```python
from build123d import *

# Parameters (mm, degrees)
ESQUISSE1_W             = 45
ESQUISSE1_H             = 45
BOSS_EXTRU_1_DEPTH      = 5
BOSS_EXTRU_2_DEPTH      = 20
BOSS_EXTRU_3_DEPTH      = 12
CONG_1_R                = 10
ESQUISSE4_W             = 4
ESQUISSE4_H             = 31.383485478
ENL_V_MAT_EXTRU_1_DEPTH = 1
ESQUISSE6_W             = 4
ESQUISSE6_H             = 28.242544177
ENL_V_MAT_EXTRU_2_DEPTH = 1
CONG_2_R                = 1
CONG_3_R                = 0.5


with BuildPart() as part:
    # Esquisse1 → Boss.-Extru.1 (new body)
    with BuildSketch(Plane.XY):
        Rectangle(ESQUISSE1_W, ESQUISSE1_H)
        with BuildLine():
            Line((14.767944635, 16.889264979), (16.889264979, 14.767944635))
            ThreePointArc((16.889264979, 14.767944635), (17.182158197, 14.060837854), (16.889264979, 13.353731073))
            Line((16.889264979, 13.353731073), (15.475051416, 11.93951751))
            ThreePointArc((15.475051416, 11.93951751), (14.828187526, 11.496881699), (14.060837854, 11.656674798))
            Line((14.060837854, 11.656674798), (11.798096154, 13.919416498))
            ThreePointArc((11.798096154, 13.919416498), (11.505202935, 14.626523279), (11.798096154, 15.33363006))
            Line((11.798096154, 15.33363006), (13.353731073, 16.889264979))
            ThreePointArc((13.353731073, 16.889264979), (14.060837854, 17.182158197), (14.767944635, 16.889264979))
        make_face(mode=Mode.SUBTRACT)
        with BuildLine():
            Line((11.93951751, -15.475051416), (13.353731073, -16.889264979))
            ThreePointArc((13.353731073, -16.889264979), (14.060837854, -17.182158197), (14.767944635, -16.889264979))
            Line((14.767944635, -16.889264979), (16.889264979, -14.767944635))
            ThreePointArc((16.889264979, -14.767944635), (17.182158197, -14.060837854), (16.889264979, -13.353731073))
            Line((16.889264979, -13.353731073), (15.33363006, -11.798096154))
            ThreePointArc((15.33363006, -11.798096154), (14.626523279, -11.505202935), (13.919416498, -11.798096154))
            Line((13.919416498, -11.798096154), (11.656674798, -14.060837854))
            ThreePointArc((11.656674798, -14.060837854), (11.496881699, -14.828187526), (11.93951751, -15.475051416))
        make_face(mode=Mode.SUBTRACT)
        with BuildLine():
            Line((-15.475051416, -11.93951751), (-16.889264979, -13.353731073))
            ThreePointArc((-16.889264979, -13.353731073), (-17.182158197, -14.060837854), (-16.889264979, -14.767944635))
            Line((-16.889264979, -14.767944635), (-14.767944635, -16.889264979))
            ThreePointArc((-14.767944635, -16.889264979), (-14.060837854, -17.182158197), (-13.353731073, -16.889264979))
            Line((-13.353731073, -16.889264979), (-11.798096154, -15.33363006))
            ThreePointArc((-11.798096154, -15.33363006), (-11.505202935, -14.626523279), (-11.798096154, -13.919416498))
            Line((-11.798096154, -13.919416498), (-14.060837854, -11.656674798))
            ThreePointArc((-14.060837854, -11.656674798), (-14.828187526, -11.496881699), (-15.475051416, -11.93951751))
        make_face(mode=Mode.SUBTRACT)
        with BuildLine():
            Line((-11.93951751, 15.475051416), (-13.353731073, 16.889264979))
            ThreePointArc((-13.353731073, 16.889264979), (-14.060837854, 17.182158197), (-14.767944635, 16.889264979))
            Line((-14.767944635, 16.889264979), (-16.889264979, 14.767944635))
            ThreePointArc((-16.889264979, 14.767944635), (-17.182158197, 14.060837854), (-16.889264979, 13.353731073))
            Line((-16.889264979, 13.353731073), (-15.33363006, 11.798096154))
            ThreePointArc((-15.33363006, 11.798096154), (-14.626523279, 11.505202935), (-13.919416498, 11.798096154))
            Line((-13.919416498, 11.798096154), (-11.656674798, 14.060837854))
            ThreePointArc((-11.656674798, 14.060837854), (-11.496881699, 14.828187526), (-11.93951751, 15.475051416))
        make_face(mode=Mode.SUBTRACT)
    extrude(amount=BOSS_EXTRU_1_DEPTH)

    # Esquisse2 → Boss.-Extru.2 (add)
    with BuildSketch(Plane.XY.offset(5)):
        Polygon((-1, 22.5), (-1, 1), (-22.5, 1), (-22.5, -1), (-1, -1), (-1, -22.5), (1, -22.5), (1, -1), (22.5, -1), (22.5, 1), (1, 1), (1, 22.5), align=None)
    extrude(amount=BOSS_EXTRU_2_DEPTH)

    # Esquisse3 → Boss.-Extru.3 (add)
    with BuildSketch(Plane(origin=(0, 0, 0), x_dir=(-1, 0, 0), z_dir=(0, 0, -1))):
        Polygon((-20.68287335, 0.883883476), (-0.883883476, 20.68287335), (20.68287335, -0.883883476), (0.883883476, -20.68287335), align=None)
    extrude(amount=BOSS_EXTRU_3_DEPTH)

    # Congé1
    cong_1_edges = [part.edges().sort_by_distance(p)[0] for p in [
        (0, 22.5, 25),
        (-22.5, 0, 25),
        (0, -22.5, 25),
        (22.5, 0, 25),
    ]]
    fillet(cong_1_edges, radius=CONG_1_R)

    # Esquisse4 → Enlèv. mat.-Extru.1 (cut)
    with BuildSketch(Plane(origin=(10.783378413, 10.783378413, 0), x_dir=(0, 0, -1), z_dir=(0.7071067811865475, 0.7071067811865477, 0))):
        with Locations((2, -1.691742739)):
            Rectangle(ESQUISSE4_W, ESQUISSE4_H)
    extrude(amount=-ENL_V_MAT_EXTRU_1_DEPTH, mode=Mode.SUBTRACT)

    # Esquisse6 → Enlèv. mat.-Extru.2 (cut)
    with BuildSketch(Plane(origin=(-10.783378413, -10.783378413, 0), x_dir=(0, 0, 1), z_dir=(-0.7071067811865476, -0.7071067811865476, 0))):
        with Locations((-2, -0.121272089)):
            Rectangle(ESQUISSE6_W, ESQUISSE6_H)
    extrude(amount=-ENL_V_MAT_EXTRU_2_DEPTH, mode=Mode.SUBTRACT)

    # Congé2
    cong_2_edges = [part.edges().sort_by_distance(p)[0] for p in [
        (9.899494937, -9.899494937, 0),
        (10.076271632, 10.076271632, 0),
        (-9.899494937, 9.899494937, 0),
        (-10.076271632, -10.076271632, 0),
    ]]
    fillet(cong_2_edges, radius=CONG_2_R)

    # Congé3
    cong_3_edges = [part.edges().sort_by_distance(p)[0] for p in [
        (10.076271632, 10.076271632, -4),
        (-10.076271632, -10.076271632, -4),
    ]]
    fillet(cong_3_edges, radius=CONG_3_R)


solid = part.part
```
Input: part model. Units: mm. Frame: model coordinates. A direction names the side the tool comes from. Coordinates: 2 decimals unless noted, no trailing zeros. Write each loop counter-clockwise with the first axis right and the second up, starting at its lowest first coordinate (ties: lowest second). Pieces come first, ordered by that corner, then holes. Notation, with made-up numbers: (-11.75, 42.25) -> (40.25, 42.25) arc R31 ccw to (40.25, 74.25) -> close; hole circle Ø7 at (72.25, 70.25). An arc over 180 degrees is marked (long way). Write each question's results on one line, items separated by ' | '.
Item 1: Material intervals for probe 1 along Z at (x, y) = (8.5, 11); probe 2 along Y at (x, z) = (9, 12); probe 3 along Y at (x, z) = (-12, 3), sorted ascending.
Conclusion:
probe 1: z = -12 to 5 | probe 2: y = -1 to 1 | probe 3: y = -22.5 to -15.54, -13.72 to 13.72, 15.54 to 22.5
Item 2: Pin query (flat end, axial travel): pin 1 Ø4 at (y, z) = (-1.5, 20.5) entering from +X; pin 2 Ø2 at (y, z) = (-3.5, 8) entering from +X; pin 3 Ø6.5 at (x, y) = (6.5, -16.5) entering from +Z. Return the tip coordinate at first contact, or that it passes through.
Conclusion:
pin 1: stops at x = 21.84 | pin 2: stops at x = 1 | pin 3: stops at z = 5
Item 3: Section query A-A on z = 11. Return loops of the section in (x, y), plus the area to 3 significant figures.
Conclusion:
outline: (-22.5, -1) -> (-1, -1) -> (-1, -22.5) -> (1, -22.5) -> (1, -1) -> (22.5, -1) -> (22.5, 1) -> (1, 1) -> (1, 22.5) -> (-1, 22.5) -> (-1, 1) -> (-22.5, 1) -> close | area: 176 mm^2
Item 4: Set-up query: faces 4 (the cylindrical face through (11.505, 14.616, 2.465)), 5 (the flat face through (-1, 12, 15)), 6 (the flat face through (-12, -12, 5)), 7 (the cylindrical face through (10.038, 10.316, -3.85)). Return all of +Z, -Z, +X, -X, +Y, -Y with unobstructed straight access to the full face (end or side cutting, diameter ignored); none if empty.
Conclusion:
face 4: +Z, -Z | face 5: +Z, -X, +Y | face 6: +Z, -X, -Y | face 7: +X, +Y
Item 5: Section query C-C on z = 19. Return loops of the section in (x, y), plus the area to 3 significant figures.
Conclusion:
outline: (-21.67, -1) -> (-1, -1) -> (-1, -21.67) -> (1, -21.67) -> (1, -1) -> (21.67, -1) -> (21.67, 1) -> (1, 1) -> (1, 21.67) -> (-1, 21.67) -> (-1, 1) -> (-21.67, 1) -> close | area: 169 mm^2
Item 6: Section query B-B on z = 4. Count the separate pieces of the cut face and the enclosed holes in it, plus the area to 3 significant figures.
Conclusion:
separate pieces: 1 | enclosed holes: 4 | area: 1,940 mm^2
Item 7: Mould query, pull axis X, two halves, no side actions, for faces 1 (the flat face through (10.922, 10.645, -7.944)), 2 (the flat face through (-12.587, -16.122, 2.465)), 3 (the flat face through (0, 22.5, 4)). Classes: +X half, -X half, draft (parallel to the pull), parting line (faces both ways), or undercut.
Conclusion:
face 1: +X half | face 2: undercut | face 3: draft
